```python
from build123d import *

# Parameters (mm, degrees)
SKETCH1_W                    = 76.2
SKETCH1_H                    = 50.8
BASE_FLANGE1_DEPTH           = 3
EDGE_FLANGE1_STRIP_W         = 18
EDGE_FLANGE1_STRIP_H         = 3
EDGE_FLANGE1_STRIP_CUT_DEPTH = 76.2
EDGE_FLANGE1_DEPTH           = 76.2
UNFOLD1_START                = -38.1
UNFOLD1_DEPTH                = 76.2
UNFOLD1_2_DEPTH              = 76.2
M5_CLEARANCE_HOLE1_D         = 5.5
M4_CLEARANCE_HOLE1_D         = 4.5
SKETCH15_R                   = 22.225
CUT_EXTRUDE1_DEPTH           = 153.340385686
M3_CLEARANCE_HOLE1_D         = 3.4
CIRPATTERN1_COUNT            = 3
SKETCH19_R                   = 11.25
CUT_EXTRUDE2_DEPTH           = 153.340385686
FOLD1_START                  = -147.468583471
FOLD1_OUTLINE_W              = 76.2
FOLD1_OUTLINE_H              = 3
FOLD1_DEPTH                  = 122.685023471
FOLD1_START_2                = -22.41644
FOLD1_2_OUTLINE_W            = 76.2
FOLD1_2_OUTLINE_H            = 124
FOLD1_2_OUTLINE_R            = 2.25
FOLD1_2_OUTLINE_R_2          = 22.225
FOLD1_2_OUTLINE_R_3          = 1.7
FOLD1_2_OUTLINE_R_4          = 11.25
FOLD1_2_DEPTH                = 0.01644
FOLD1_START_3                = -25.4
FOLD1_3_OUTLINE_W            = 76.2
FOLD1_3_OUTLINE_H            = 124
FOLD1_3_OUTLINE_R            = 2.25
FOLD1_3_OUTLINE_R_2          = 22.225
FOLD1_3_OUTLINE_R_3          = 1.7
FOLD1_3_OUTLINE_R_4          = 11.25
FOLD1_3_DEPTH                = 6
FOLD1_START_4                = -38.1
FOLD1_4_DEPTH                = 76.2


with BuildPart() as part:
    # Base-Flange1: sheet metal written as solids
    # Sketch1 → Base-Flange1 (new body)
    with BuildSketch(Plane(origin=(0, 0, 0), x_dir=(1, 0, 0), z_dir=(0, 1, 0))):
        Rectangle(SKETCH1_W, SKETCH1_H)
    extrude(amount=-BASE_FLANGE1_DEPTH)

    # Edge-Flange1: sheet metal written as solids
    # Edge-Flange1 strip (on a plane across the edge) → Edge-Flange1 strip cut (cut)
    with BuildSketch(Plane(origin=(38.1, 0, -25.4), x_dir=(0, 0, 1), z_dir=(-1, 0, 0))):
        with Locations((-3, -1.5)):
            Rectangle(EDGE_FLANGE1_STRIP_W, EDGE_FLANGE1_STRIP_H)
    extrude(amount=EDGE_FLANGE1_STRIP_CUT_DEPTH, mode=Mode.SUBTRACT)

    # Edge-Flange1 section (on a plane across the edge) → Edge-Flange1 (add)
    with BuildSketch(Plane(origin=(38.1, 0, -25.4), x_dir=(0, 0, 1), z_dir=(-1, 0, 0))):
        with BuildLine():
            Line((0, 3), (0, 124))
            Line((0, 124), (3, 124))
            Line((3, 124), (3, 3))
            ThreePointArc((3, 3), (3.878679656, 0.878679656), (6, 0))
            Line((6, 0), (6, -3))
            ThreePointArc((6, -3), (1.757359313, -1.242640687), (0, 3))
        make_face()
    extrude(amount=EDGE_FLANGE1_DEPTH)

    # Unfold1: read off the stored shape, not the designer's step
    # Unfold1 outline → Unfold1 (cut)
    with BuildSketch(Plane.YZ.offset(UNFOLD1_START)):
        with BuildLine():
            Line((0, -19.4), (0, -24.596152423))
            ThreePointArc((0, -24.596152423), (1.447085729, -25.195554958), (3, -25.4))
            Line((3, -25.4), (124, -25.4))
            Line((124, -25.4), (124, -22.4))
            Line((124, -22.4), (3, -22.4))
            ThreePointArc((3, -22.4), (0.878679656, -21.521320344), (0, -19.4))
        make_face()
    extrude(amount=UNFOLD1_DEPTH, mode=Mode.SUBTRACT)

    # Unfold1 2 outline → Unfold1 2 (add)
    with BuildSketch(Plane.YZ.offset(UNFOLD1_START)):
        with BuildLine():
            Line((-3, -19.4), (-3, -147.468583471))
            Line((-3, -147.468583471), (0, -147.468583471))
            Line((0, -147.468583471), (0, -24.596152423))
            ThreePointArc((0, -24.596152423), (-2.196152423, -22.4), (-3, -19.4))
        make_face()
    extrude(amount=UNFOLD1_2_DEPTH)

    # M5 Clearance Hole1 (through all)
    with Locations(Plane(origin=(0, 0, 0), x_dir=(1, 0, 0), z_dir=(0, 1, 0))):
        with Locations((-25.4, 12.7), (-25.4, -12.7), (25.4, -12.7), (25.4, 12.7)):
            Hole(M5_CLEARANCE_HOLE1_D / 2)

    # M4 Clearance Hole1 (through all)
    with Locations(Plane(origin=(0, 0, 0), x_dir=(1, 0, 0), z_dir=(0, 1, 0))):
        with Locations((-23.5, 41.418583471), (23.5, 88.418583471), (-23.5, 88.418583471), (23.5, 41.418583471)):
            Hole(M4_CLEARANCE_HOLE1_D / 2)

    # Sketch15 → Cut-Extrude1 (cut, through all)
    with BuildSketch(Plane(origin=(0, 0, 0), x_dir=(1, 0, 0), z_dir=(0, 1, 0))):
        with Locations(Location((0, 64.918583471, 0), (0, 0, 270))):
            Circle(SKETCH15_R)
    extrude(amount=-CUT_EXTRUDE1_DEPTH, mode=Mode.SUBTRACT)

    # M3 Clearance Hole1 (through all)
    with Locations(Plane(origin=(0, 0, 0), x_dir=(1, 0, 0), z_dir=(0, 1, 0))):
        with Locations((0, 136.068583471), (-7.5, 135.058964527)):
            m3_clearance_hole1 = Hole(M3_CLEARANCE_HOLE1_D / 2)

    # CirPattern1: M3 Clearance Hole1 ×3 about axis
    cirpattern1_axis = Axis((0, 0, -122.068583471), (0, 1, 0))
    for i in range(1, CIRPATTERN1_COUNT):
        add(m3_clearance_hole1.rotate(cirpattern1_axis, i * 360 / CIRPATTERN1_COUNT), mode=Mode.SUBTRACT)

    # Sketch19 → Cut-Extrude2 (cut, through all)
    with BuildSketch(Plane(origin=(0, 0, 0), x_dir=(1, 0, 0), z_dir=(0, 1, 0))):
        with Locations(Location((0, 122.068583471, 0), (0, 0, 270))):
            Circle(SKETCH19_R)
        with BuildLine():
            Line((-25.4, 102.512292942), (25.4, 102.512292942))
            ThreePointArc((25.4, 102.512292942), (28.6639, 99.248392942), (25.4, 95.984492942))
            Line((25.4, 95.984492942), (-25.4, 95.984492942))
            ThreePointArc((-25.4, 95.984492942), (-28.6639, 99.248392942), (-25.4, 102.512292942))
        make_face()
    extrude(amount=-CUT_EXTRUDE2_DEPTH, mode=Mode.SUBTRACT)

    # Fold1: read off the stored shape, not the designer's step
    # Fold1 outline → Fold1 (cut)
    with BuildSketch(Plane.XY.offset(FOLD1_START)):
        with Locations((0, -1.5)):
            Rectangle(FOLD1_OUTLINE_W, FOLD1_OUTLINE_H)
    extrude(amount=FOLD1_DEPTH, mode=Mode.SUBTRACT)

    # Fold1 2 outline → Fold1 2 (add)
    with BuildSketch(Plane.XY.offset(FOLD1_START_2)):
        with Locations((0, 62)):
            Rectangle(FOLD1_2_OUTLINE_W, FOLD1_2_OUTLINE_H)
        with Locations((-23.5, 17.95)):
            Circle(FOLD1_2_OUTLINE_R, mode=Mode.SUBTRACT)
        with Locations((23.5, 17.95)):
            Circle(FOLD1_2_OUTLINE_R, mode=Mode.SUBTRACT)
        with Locations((0, 41.45)):
            Circle(FOLD1_2_OUTLINE_R_2, mode=Mode.SUBTRACT)
        with Locations((-23.5, 64.95)):
            Circle(FOLD1_2_OUTLINE_R, mode=Mode.SUBTRACT)
        with Locations((-12.124355653, 91.6)):
            Circle(FOLD1_2_OUTLINE_R_3, mode=Mode.SUBTRACT)
        with Locations((-7.5, 85.609618943)):
            Circle(FOLD1_2_OUTLINE_R_3, mode=Mode.SUBTRACT)
        with Locations((-7.5, 111.590381057)):
            Circle(FOLD1_2_OUTLINE_R_3, mode=Mode.SUBTRACT)
        with BuildLine():
            ThreePointArc((-25.4, 72.515909472), (-28.6639, 75.779809472), (-25.4, 79.043709472))
            Line((-25.4, 79.043709472), (25.4, 79.043709472))
            ThreePointArc((25.4, 79.043709472), (28.6639, 75.779809472), (25.4, 72.515909472))
            Line((25.4, 72.515909472), (-25.4, 72.515909472))
        make_face(mode=Mode.SUBTRACT)
        with Locations((12.124355653, 91.6)):
            Circle(FOLD1_2_OUTLINE_R_3, mode=Mode.SUBTRACT)
        with Locations((23.5, 64.95)):
            Circle(FOLD1_2_OUTLINE_R, mode=Mode.SUBTRACT)
        with Locations((0, 98.6)):
            Circle(FOLD1_2_OUTLINE_R_4, mode=Mode.SUBTRACT)
        with Locations((15, 98.6)):
            Circle(FOLD1_2_OUTLINE_R_3, mode=Mode.SUBTRACT)
        with Locations((0, 112.6)):
            Circle(FOLD1_2_OUTLINE_R_3, mode=Mode.SUBTRACT)
    extrude(amount=FOLD1_2_DEPTH)

    # Fold1 3 outline → Fold1 3 (add)
    with BuildSketch(Plane.XY.offset(FOLD1_START_3)):
        with Locations((0, 62)):
            Rectangle(FOLD1_3_OUTLINE_W, FOLD1_3_OUTLINE_H)
        with Locations((-23.5, 17.95)):
            Circle(FOLD1_3_OUTLINE_R, mode=Mode.SUBTRACT)
        with Locations((23.5, 17.95)):
            Circle(FOLD1_3_OUTLINE_R, mode=Mode.SUBTRACT)
        with Locations((0, 41.45)):
            Circle(FOLD1_3_OUTLINE_R_2, mode=Mode.SUBTRACT)
        with Locations((-23.5, 64.95)):
            Circle(FOLD1_3_OUTLINE_R, mode=Mode.SUBTRACT)
        with Locations((-12.124355653, 91.6)):
            Circle(FOLD1_3_OUTLINE_R_3, mode=Mode.SUBTRACT)
        with Locations((-7.5, 85.609618943)):
            Circle(FOLD1_3_OUTLINE_R_3, mode=Mode.SUBTRACT)
        with Locations((-7.5, 111.590381057)):
            Circle(FOLD1_3_OUTLINE_R_3, mode=Mode.SUBTRACT)
        with BuildLine():
            ThreePointArc((-25.4, 72.515909472), (-28.6639, 75.779809472), (-25.4, 79.043709472))
            Line((-25.4, 79.043709472), (25.4, 79.043709472))
            ThreePointArc((25.4, 79.043709472), (28.6639, 75.779809472), (25.4, 72.515909472))
            Line((25.4, 72.515909472), (-25.4, 72.515909472))
        make_face(mode=Mode.SUBTRACT)
        with Locations((12.124355653, 91.6)):
            Circle(FOLD1_3_OUTLINE_R_3, mode=Mode.SUBTRACT)
        with Locations((23.5, 64.95)):
            Circle(FOLD1_3_OUTLINE_R, mode=Mode.SUBTRACT)
        with Locations((0, 98.6)):
            Circle(FOLD1_3_OUTLINE_R_4, mode=Mode.SUBTRACT)
        with Locations((15, 98.6)):
            Circle(FOLD1_3_OUTLINE_R_3, mode=Mode.SUBTRACT)
        with Locations((0, 112.6)):
            Circle(FOLD1_3_OUTLINE_R_3, mode=Mode.SUBTRACT)
    extrude(amount=FOLD1_3_DEPTH)

    # Fold1 4 outline → Fold1 4 (cut)
    with BuildSketch(Plane.YZ.offset(FOLD1_START_4)):
        with BuildLine():
            Line((124, -22.4), (124, -19.4))
            Line((124, -19.4), (0, -19.4))
            ThreePointArc((0, -19.4), (0.878679656, -21.521320344), (3, -22.4))
            Line((3, -22.4), (124, -22.4))
        make_face()
        with BuildLine():
            Line((0, -25.4), (3, -25.4))
            ThreePointArc((3, -25.4), (-1.242640687, -23.642640687), (-3, -19.4))
            Line((-3, -19.4), (-3, -24.78356))
            Line((-3, -24.78356), (0, -24.78356))
            Line((0, -24.78356), (0, -25.4))
        make_face()
    extrude(amount=FOLD1_4_DEPTH, mode=Mode.SUBTRACT)


solid = part.part
```
Geometry: final body of the model. Coordinates: model frame, mm. A direction names the side the tool comes from. Round coordinates to 2 decimals unless told otherwise and drop trailing zeros. Write each loop counter-clockwise with the first axis right and the second up, starting at its lowest first coordinate (ties: lowest second). Pieces come first, ordered by that corner, then holes. Notation, with made-up numbers: (33.25, 58.5) -> (92.25, 58.5) arc R16 cw to (92.25, 75.5) -> close; hole circle Ø6 at (75, 9.25). An arc over 180 degrees is marked (long way). Use CSV: the item, a comma, the result in double quotes. Start each with the question number.
Q1. Pull-direction query (Z, two-part tool) for faces 1 (the face through (-9, 63, -22.4)), 2 (the face through (-23.218, -1.521, 14.373)), 3 (the face through (-2.893, 63.486, -23.921)); classes: pulls with the +Z half, pulls with the -Z half, needs draft (parallel to the pull), parting line crosses it, or undercut.
Q2. Section B-B (z = -12.7). Return loops of the section in (x, y), plus the area to 3 significant figures.
Q3. Section C-C (x = -17). Return loops of the section in (y, z), plus the area to 3 significant figures.
Q4. Line query: L1, parallel to X at y = -1.2, z = -12.7; L2, parallel to X at y = 64.95, z = -23.05; L3, parallel to Y at x = 15, z = -23.2. Output: solid intervals per line, ascending.
Q5. Reachability of faces 4 (the face through (-1, 0, 3)), 5 (the face through (-28.663, 75.708, -23.921)), 6 (the face through (22.78, -1.52, -13.53)) from +Z, -Z, +X, -X, +Y, -Y: full face, straight path, thin tool, end or side. Return the list, or none.
Q6. First-contact query: pin 1 Ø7 at (x, y) = (-23.5, 64.95) entering from +Z; pin 2 Ø22.5 at (x, z) = (-3, -4) entering from +Y. Flat tips, straight axial feed; report the tip coordinate or a pass-through.
Q7. Section A-A (x = 0). Return loops of the section in (y, z) (3 decimals), plus the area to 3 significant figures.
Q8. Section D-D (y = 91.6). Return loops of the section in (x, z).
Result sheet:
1,face 1,"pulls with the +Z half"
1,face 2,"undercut"
1,face 3,"needs draft"
2,outline,"(-38.1, -3) -> (-28.15, -3) -> (-28.15, 0) -> (-38.1, 0) -> close; (-22.65, -3) -> (22.65, -3) -> (22.65, 0) -> (-22.65, 0) -> close; (28.15, -3) -> (38.1, -3) -> (38.1, 0) -> (28.15, 0) -> close"
2,area,"196 mm²"
3,outline,"(-3, -19.4) arc R6 ccw to (3, -25.4) -> (27.13, -25.4) -> (27.13, -22.4) -> (3, -22.4) arc R3 cw to (0, -19.4) -> (0, 25.4) -> (-3, 25.4) -> close; (55.77, -25.4) -> (72.52, -25.4) -> (72.52, -22.4) -> (55.77, -22.4) -> close; (79.04, -25.4) -> (124, -25.4) -> (124, -22.4) -> (79.04, -22.4) -> close"
3,area,"413 mm²"
4,L1,"-38.1 to -28.15, -22.65 to 22.65, 28.15 to 38.1"
4,L2,"-38.1 to -25.75, -21.25 to 21.25, 25.75 to 38.1"
4,L3,"-1.64 to 25.05, 57.85 to 72.52, 79.04 to 96.9, 100.3 to 124"
5,face 4,"+Z, +X, -X, +Y"
5,face 5,"+Z, -Z"
5,face 6,"+Y, -Y"
6,pin 1,"z = -22.4"
6,pin 2,"y = 0"
7,outline,"(-3, -19.4) arc R6 ccw to (3, -25.4) -> (19.225, -25.4) -> (19.225, -22.4) -> (3, -22.4) arc R3 cw to (0, -19.4) -> (0, 25.4) -> (-3, 25.4) -> close; (63.675, -25.4) -> (72.516, -25.4) -> (72.516, -22.4) -> (63.675, -22.4) -> close; (79.044, -25.4) -> (87.35, -25.4) -> (87.35, -22.4) -> (79.044, -22.4) -> close; (109.85, -25.4) -> (110.9, -25.4) -> (110.9, -22.4) -> (109.85, -22.4) -> close; (114.3, -25.4) -> (124, -25.4) -> (124, -22.4) -> (114.3, -22.4) -> close"
7,area,"288 mm²"
8,outline,"(-38.1, -25.4) -> (-13.82, -25.4) -> (-13.82, -22.4) -> (-38.1, -22.4) -> close; (-10.42, -25.4) -> (-8.81, -25.4) -> (-8.81, -22.4) -> (-10.42, -22.4) -> close; (8.81, -25.4) -> (10.42, -25.4) -> (10.42, -22.4) -> (8.81, -22.4) -> close; (13.82, -25.4) -> (38.1, -25.4) -> (38.1, -22.4) -> (13.82, -22.4) -> close"
